Here's how the part is built. I have some questions about the finished solid (model axes, mm). A direction names the side the tool comes from. Round coordinates to 2 decimals unless told otherwise and drop trailing zeros. Order: outer loops, then holes, each group sorted by start corner. A loop starts at its lowest first (then second) coordinate and runs counter-clockwise, first axis right, second up.
Autodesk Inventor part; units mm, degrees
ref_plane "YZ Plane" through (0, 0, 0) normal (1, 0, 0) x (0, 1, 0)
ref_plane "XZ Plane" through (0, 0, 0) normal (0, 1, 0) x (-1, 0, 0)
ref_plane "XY Plane" through (0, 0, 0) normal (0, 0, 1) x (1, 0, 0)
sketch "Sketch1" plane through (0, 0, 0) normal (0, 1, 0) x (-1, 0, 0)
  line L0 (0, 0) -> (180, 0)
  line L1 (180, 0) -> (180, -140)
  line L2 (180, -140) -> (0, -140)
  line L3 (0, -140) -> (0, 0)
  line L4 (0, 0) -> (0, -10)
  line L5 (0, -10) -> (10, -10)
  line L6 (180, -140) -> (170, -140)
  line L7 (170, -140) -> (170, -130)
  line L8 (170, -130) -> (10, -130)
  line L9 (10, -130) -> (10, -10)
  line L10 (10, -10) -> (170, -10)
  line L11 (170, -10) -> (170, -130)
  line L12 (90, -130) -> (95, -130)
  line L13 (95, -130) -> (85, -130)
  line L14 (85, -130) -> (85, -10)
  line L15 (85, -10) -> (95, -10)
  line L16 (95, -10) -> (95, -130)
  line L17 (170, -70) -> (170, -75)
  line L18 (170, -75) -> (10, -75)
  line L19 (10, -75) -> (10, -65)
  line L20 (10, -65) -> (170, -65)
  line L21 (170, -65) -> (170, -75)
  dimension "d0" = 180
  dimension "d1" = 140
  dimension "d2" = 10
  dimension "d3" = 10
  dimension "d4" = 10
  dimension "d5" = 10
  dimension "d6" = 5
  dimension "d7" = 10
  dimension "d8" = 5
  dimension "d9" = 10
extrude "Extrusion1" add sketch "Sketch1" along normal blind 10 contours L0 L1 L2 L7 L11 L10 L5 L3 | L5 L9 L8 L7 L2 L3 | L20 L14 L18 L9 | L10 L16 L20 L14 | L20 L16 L18 L14 | L8 L14 L18 L16 | L18 L16 L20 L11
sketch "Sketch2" plane through (0, 0, -140) normal (0, 0, -1) x (-1, 0, 0)
  line L0 (180, 0) -> (0, 0)
  line L1 (170, 0) -> (170, 10)
  line L2 (180, 0) -> (170, 0)
  line L3 (170, 0) -> (170, 10)
  line L4 (170, 10) -> (180, 10)
  line L5 (180, 10) -> (180, 0)
  line L6 (10, 0) -> (10, 10)
  line L7 (0, 0) -> (10, 0)
  line L8 (10, 0) -> (10, 10)
  line L9 (10, 10) -> (0, 10)
  line L10 (0, 10) -> (0, 0)
  dimension "d12" = 10
  dimension "d13" = 10
  dimension "d14" = 10
extrude "Extrusion2" add sketch "Sketch2" along normal blind 20
sketch "Sketch3" plane through (-180, 0, 0) normal (0, 0, 1) x (1, 0, 0)
  line L0 (0, 10) -> (10, 10)
  line L1 (85, 0) -> (10, 0)
  line L2 (0, 10) -> (10, 10)
  line L3 (10, 10) -> (10, 0)
  line L4 (10, 0) -> (0, 0)
  line L5 (0, 0) -> (0, 10)
  line L6 (180, 0) -> (180, 10)
  line L7 (170, 0) -> (95, 0)
  line L8 (180, 10) -> (170, 10)
  line L9 (170, 10) -> (170, 0)
  line L10 (170, 0) -> (180, 0)
  line L11 (180, 0) -> (180, 10)
  dimension "d17" = 10
extrude "Extrusion3" add sketch "Sketch3" along normal blind 20
sketch "Sketch4" plane through (0, 10, 0) normal (0, 1, 0) x (1, 0, 0)
  line L0 (-180, -20) -> (-180, 160)
  line L1 (-170, 0) -> (-170, -20)
  line L2 (-180, -20) -> (-170, -20)
  line L3 (-170, -20) -> (-170, -10)
  line L4 (-170, -10) -> (-180, -10)
  line L5 (-180, -10) -> (-180, -20)
  line L6 (-170, 140) -> (-170, 160)
  line L7 (-180, 160) -> (-170, 160)
  line L8 (-170, 160) -> (-170, 150)
  line L9 (-170, 150) -> (-180, 150)
  line L10 (-180, 150) -> (-180, 160)
  line L11 (-10, 160) -> (0, 160)
  line L12 (0, 160) -> (0, -20)
  line L13 (-10, 160) -> (0, 160)
  line L14 (0, 160) -> (0, 150)
  line L15 (0, 150) -> (-10, 150)
  line L16 (-10, 150) -> (-10, 160)
  line L17 (-10, -20) -> (0, -20)
  line L18 (-10, 0) -> (-10, -20)
  line L19 (0, -20) -> (-10, -20)
  line L20 (-10, -20) -> (-10, -15)
  line L21 (0, -15) -> (0, -20)
  line L22 (0, -20) -> (0, 160)
  line L23 (-10, 0) -> (-10, -20)
  line L24 (0, -20) -> (-10, -20)
  line L25 (-10, -20) -> (-10, -10)
  line L26 (-10, -10) -> (0, -10)
  line L27 (0, -10) -> (0, -20)
  point P0 (0, 0)
  dimension "d20" = 10
  dimension "d21" = 10
  dimension "d22" = 10
  dimension "d50" = 10
extrude "Extrusion4" add sketch "Sketch4" along normal blind 80
sketch "Sketch7" plane through (0, 90, 0) normal (0, 1, 0) x (1, 0, 0)
  line L0 (-10, -20) -> (0, -20)
  line L1 (-5, -20) -> (-5, -15)
  line L2 (0, 160) -> (-10, 160)
  line L3 (-5, 160) -> (-5, 155)
  circle A0 centre (-5, 155) radius 2.4
  circle A1 centre (-5, -15) radius 2.4
  circle A2 centre (-175, 155) radius 2.4
  circle A3 centre (-175, -15) radius 2.4
  point P0 (0, 0)
  dimension "d40" = 5
  dimension "d41" = 5
  dimension "d42" = 4.8
  dimension "d47" = 4.8
  dimension "d51" = 4.8
  dimension "d52" = 4.8
extrude "Extrusion7" cut sketch "Sketch7" against normal blind 25
properties part number "Raket_Holder"
1. I'm going to push flat-ended pins straight in: P1, Ø3, axis at x = -43.5, y = 5, coming from the -Z side; P2, Ø5, axis at x = -144.5, y = 7, coming from the +Z side; P3, Ø3, axis at x = -175, z = 15, coming from the +Y side. Where does each tip first touch, or does it pass through?
Evaluation:
P1: stops at z = -140
P2: stops at z = 0
P3: stops at y = 65
2. If we section it at A-A, the plane y = 32.5: Write out the boundary of the cut face in (x, z), and give its area (3 significant figures).
Evaluation:
outline: (-180, -160) - (-170, -160) - (-170, -150) - (-180, -150) - close; (-180, 10) - (-170, 10) - (-170, 20) - (-180, 20) - close; (-10, -160) - (0, -160) - (0, -150) - (-10, -150) - close; (-10, 10) - (0, 10) - (0, 20) - (-10, 20) - close
area: 400 mm2
3. If we mould it in two halves opening along Z, with no side actions, what happens to faces 1 (the flat face through (-48, 5, -130)), 2 (the flat face through (-10, 44, -154)), 3 (the flat face through (-91, 5, -140)), 4 (the flat face through (-85, 5, -103))? For each: released by +Z, released by -Z, zero draft, split by the parting line, or undercut.
Evaluation:
face 1: undercut
face 2: zero draft
face 3: released by -Z
face 4: undercut
4. If we section it at B-B, the plane x = -105.5: Write out the boundary of the cut face in (y, z).
Evaluation:
outline: (0, -140) - (10, -140) - (10, -130) - (0, -130) - close; (0, -75) - (10, -75) - (10, -65) - (0, -65) - close; (0, -10) - (10, -10) - (10, 0) - (0, 0) - close
5. On a 3-axis mill with a long thin cutter (end or side, diameter ignored), from which of +Z, -Z, +X, -X, +Y, -Y can I reach the whole of each face in a straight line? I mean faces 5 (the flat face through (-89, 5, 0)), 6 (the cylindrical face through (-172.783, 77.675, 15.919)), 7 (the flat face through (-10, 5, -38)), 8 (the flat face through (-175, 49, 10)). Say none if no direction works.
Evaluation:
face 5: +Z, +Y, -Y
face 6: +Y
face 7: +Y, -Y
face 8: +X, -X, +Y
6. If we section it at C-C, the plane z = -62.5: Write out the boundary of the cut face in (x, y).
Evaluation:
outline: (-180, 0) - (-170, 0) - (-170, 10) - (-180, 10) - close; (-95, 0) - (-85, 0) - (-85, 10) - (-95, 10) - close; (-10, 0) - (0, 0) - (0, 10) - (-10, 10) - close
7. I need wall thicknesses on probe 1 along Z at (x, y) = (-5, 75); probe 2 along X at (y, z) = (71.5, 15); probe 3 along X at (y, z) = (4, -121.5). Which ranges of each line are inside material? Lowest first, please.
Evaluation:
probe 1: z = -160 to -157.4, -152.6 to -150, 10 to 12.6, 17.4 to 20
probe 2: x = -180 to -177.4, -172.6 to -170, -10 to -7.4, -2.6 to 0
probe 3: x = -180 to -170, -95 to -85, -10 to 0
8. If we section it at D-D, the plane y = 68: Write out the boundary of the cut face in (x, z), and give its area (3 significant figures).
Evaluation:
outline: (-180, -160) - (-170, -160) - (-170, -150) - (-180, -150) - close; (-180, 10) - (-170, 10) - (-170, 20) - (-180, 20) - close; (-10, -160) - (0, -160) - (0, -150) - (-10, -150) - close; (-10, 10) - (0, 10) - (0, 20) - (-10, 20) - close; hole circle Ø4.8 at (-175, -155); hole circle Ø4.8 at (-175, 15); hole circle Ø4.8 at (-5, -155); hole circle Ø4.8 at (-5, 15)
area: 328 mm2
